The listing builds one solid part. Answer for the finished solid, in the listing's coordinates (mm). A direction names the side the tool comes from. Give positions to 0.01 mm unless a question says otherwise; leave off trailing zeros. Loops run counter-clockwise (first coordinate to the right, second up) from the corner with the lowest first, then second, coordinate; pieces in that order, holes last. Notation, with made-up numbers: (5, 76) - (17, 76) arc R15 cw to (17, 93) - close; hole circle Ø1 at (40, 77.5). An arc over 180 degrees is marked (long way). One line per item, written item: value. Start each with the question number.
from build123d import *

# Parameters (mm, degrees)
F0_W       = 1371.6
F0_H       = 609.6
F1_DEPTH   = 254
F2_W       = 926.5377521515
F2_H       = 609.6
F1_FACE1_W = 1371.6
F1_FACE1_H = 609.6
F3_DEPTH   = 1522.3157249


# Not quite as in the source:
# - an extrude ends at something that could not be found from the text; its depth is read off the source's solid


with BuildPart() as f1:
    # F0 (on Top) → F1 (new body)
    with BuildSketch(Plane.XY):
        with Locations((54.0854626386, 40.4904214665)):
            Rectangle(F0_W, F0_H)
    extrude(amount=F1_DEPTH)

    # F2 (on face) + F1_face1 (on face) → F3 (join, through all)
    with BuildSketch(Plane.XY.offset(254)):
        with Locations((71.9089508057, 40.4904214665)):
            Rectangle(F2_W, F2_H)
    with BuildSketch(Plane(origin=(54.0854626386, 40.4904214665, 0), x_dir=(1, 0, 0), z_dir=(0, 0, -1))):
        Rectangle(F1_FACE1_W, F1_FACE1_H)
    extrude(amount=F3_DEPTH, dir=(0, 0, 1))


solid = f1.part
1. Find the intervals of material crossed by L1, parallel to Z at x = 657, y = -111; L2, parallel to X at y = -202, z = 1664, in increasing order. Write a range as [from, to].
2. A cutting plane is placed at B-B (x = 606.5). Determine the outline of the cut face in (y, z), plus the area to 3 significant figures.
3. A flat-ended cylindrical pin translates along its axis: pin 1 (8 mm diameter, centred on x = 569.5, y = -39.5, fed in from -Z). Find the tip coordinate at first contact, or state that the pin passes through.
4. For faces 1 (the flat face through (-513, 36, 1522.316)), 2 (the flat face through (535.178, 36, 1648)), 3 (the flat face through (44, 45, 0)), determine the directions among +Z, -Z, +X, -X, +Y, -Y from which every point of the face is accessible in a straight line to the end or side of a thin tool.
5. A cutting plane is placed at C-C (z = 1555). Determine the outline of the cut face in (x, y).
6. A cutting plane is placed at A-A (y = 248). Determine the outline of the cut face in (x, z), plus the area to 3 significant figures.
Results below:
1. L1: z = [0, 1522.32]
1. L2: x = [-391.36, 535.18]
2. outline: (-264.31, 0) - (345.29, 0) - (345.29, 1522.32) - (-264.31, 1522.32) - close
2. area: 928,000 mm^2
3. pin 1: stops at z = 0
4. face 1: +Z, -X, +Y, -Y
4. face 2: +Z, +X, +Y, -Y
4. face 3: -Z, +X, -X, +Y, -Y
5. outline: (-391.36, -264.31) - (535.18, -264.31) - (535.18, 345.29) - (-391.36, 345.29) - close
6. outline: (-631.71, 0) - (739.89, 0) - (739.89, 1522.32) - (535.18, 1522.32) - (535.18, 1776.32) - (-391.36, 1776.32) - (-391.36, 1522.32) - (-631.71, 1522.32) - close
6. area: 2,320,000 mm^2
